Source: three-view drawing plus pictorial views. Frame: mm from the lowest corner of the part. Round coordinates to 2 decimals unless told otherwise and drop trailing zeros. Order: outer loops, then holes, each group sorted by start corner. A loop starts at its lowest first (then second) coordinate and runs counter-clockwise, first axis right, second up. Notation, with made-up numbers: (42, 73) -> (48, 73) arc R16 cw to (48, 83) -> close; hole circle Ø2 at (82.5, 23.5). An arc over 180 degrees is marked (long way). Answer as CSV lines item,"result". Start each with the question number.
1) First-contact query: P1, Ø5, axis at y = 27, z = 6.5, coming from the +X side; P2, Ø1, axis at x = 122, y = 13, coming from the +Z side; P3, Ø8, axis at y = 17.5, z = 23, coming from the -X side. Flat tips, straight axial feed; report the tip coordinate or a pass-through.
2) Section query D-D, the plane y = 5. Output: boundary loops of the cut face in (x, z) (1 decimal).
3) Section query A-A, the plane y = 12.5. Output: boundary loops of the cut face in (x, z) (1 decimal).
4) Line query: L1, parallel to Z at x = 22.5, y = 32.5; L2, parallel to X at y = 28, z = 7.5 (1 decimal); L3, parallel to Y at x = 81.5, z = 2 (1 decimal). Output: solid intervals per line, ascending.
5) Section query C-C, the plane z = 23.25. Output: boundary loops of the cut face in (x, y) (1 decimal).
6) Section query B-B, the plane x = 44.5. Output: boundary loops of the cut face in (y, z) (1 decimal).
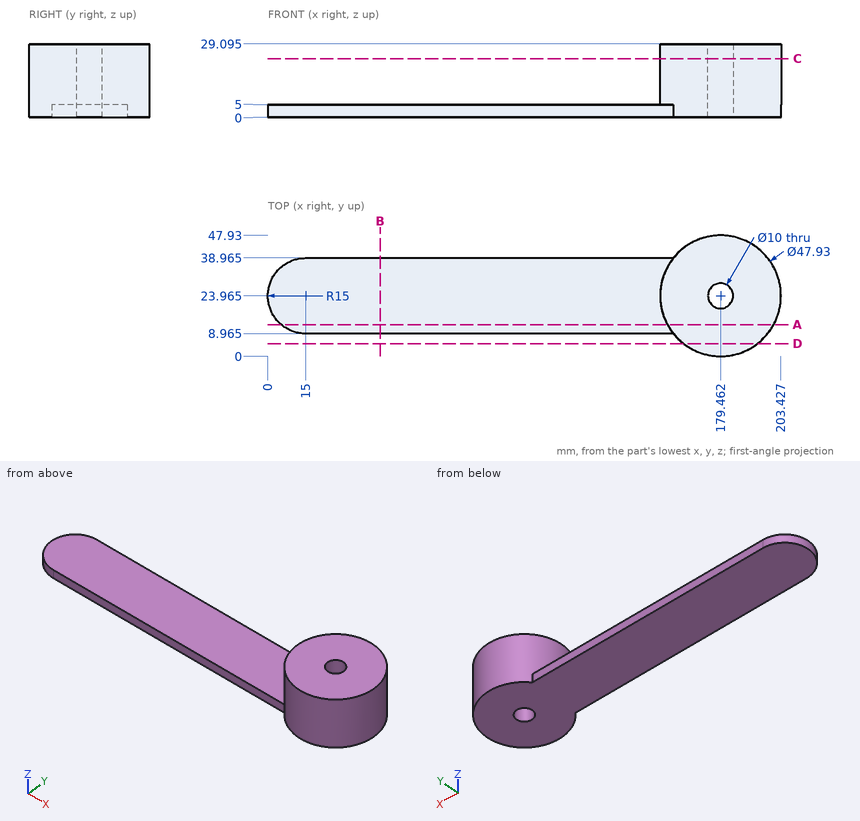
Findings:
1,P1,"stops at x = 203.42"
1,P2,"stops at z = 5"
1,P3,"stops at x = 155.62"
2,outline,"(164.8, 0) -> (194.1, 0) -> (194.1, 29.1) -> (164.8, 29.1) -> close"
3,outline,"(5.3, 0) -> (200.5, 0) -> (200.5, 29.1) -> (158.4, 29.1) -> (158.4, 5) -> (5.3, 5) -> close"
4,L1,"z = 0 to 5"
4,L2,"x = 155.8 to 176.5, 182.4 to 203.1"
4,L3,"y = 9 to 39"
5,outline,"circle Ø47.9 at (179.5, 24); hole circle Ø10 at (179.5, 24)"
6,outline,"(9, 0) -> (39, 0) -> (39, 5) -> (9, 5) -> close"
